Input: part model. Units: mm. Frame: model coordinates. Round coordinates to 2 decimals unless told otherwise and drop trailing zeros. Write each loop counter-clockwise with the first axis right and the second up, starting at its lowest first coordinate (ties: lowest second). Pieces come first, ordered by that corner, then holes. Notation, with made-up numbers: (-6, 40) - (29, 40) arc R12 cw to (29, 46) - close; hole circle Ø9 at (-12, 49.25). An arc over 180 degrees is marked (long way). Use one line per item in the form item = value.
Solid Edge part; units mm, degrees
sketch "Sketch1" plane through (0, 0, 0) normal (1, 0, 0) x (0, 1, 0)
  circle A0 centre (0, 0) radius 5
extrude "Protrusion1" add sketch "Sketch1" along normal mid plane 55
cosmetic_thread "Thread_1" thread depth 15
cosmetic_thread "Thread_2" thread depth 18
sketch "Sketch2" plane through (0, 0, 0) normal (0, 0, 1) x (1, 0, 0)
  circle A0 centre (-23.5, 0) radius 1.4
  circle A1 centre (23.5, 0) radius 1.25
extrude "ExtrudedCutout_1" cut sketch "Sketch2" along normal mid plane 31.5098
(1) Draft query along X for faces 1 (the face through (-27.5, 0, 0)), 2 (the face through (27.5, 0, 0)), 3 (the face through (24.655, 0.479, -0.07)). Return one class per face: released by +X, released by -X, zero draft, split by the parting line, or undercut.
Derived:
face_1 = released by -X
face_2 = released by +X
face_3 = undercut
(2) Cut plane D-D on x = -8. Output: boundary loops of the cut face in (y, z).
Derived:
outline = circle Ø10 at (0, 0)
(3) First-contact query: pin 1 Ø1.5 at (x, y) = (3.5, -2) entering from -Z; pin 2 Ø6 at (x, y) = (5.5, -3) entering from +Z; pin 3 Ø1.5 at (x, z) = (-12, -2.5) entering from -Y; pin 4 Ø3 at (x, y) = (-19, 2.5) entering from +Z. Flat tips, straight axial feed; report the tip coordinate or a pass-through.
Derived:
pin_1 = -4.84
pin_2 = 5
pin_3 = -4.68
pin_4 = 4.9
(4) Cut plane B-B on z = 0. Output: boundary loops of the cut face in (x, y).
Derived:
outline = (-27.5, -5) - (27.5, -5) - (27.5, 5) - (-27.5, 5) - close; hole circle Ø2.8 at (-23.5, 0); hole circle Ø2.5 at (23.5, 0)
(5) Cut plane A-A on y = 0. Output: boundary loops of the cut face in (x, z), then the cut area to 3 significant figures.
Derived:
outline = (-27.5, -5) - (-24.9, -5) - (-24.9, 5) - (-27.5, 5) - close; (-22.1, -5) - (22.25, -5) - (22.25, 5) - (-22.1, 5) - close; (24.75, -5) - (27.5, -5) - (27.5, 5) - (24.75, 5) - close
area = 497 mm^2
(6) Cut plane C-C on x = -23.5. Output: boundary loops of the cut face in (y, z).
Derived:
outline = (-1.4, -4.8) - (-1.4, 4.8) arc R5 ccw to start; (1.4, -4.8) arc R5 ccw to (1.4, 4.8) - close
(7) Material intervals for L1, parallel to X at y = 0, z = 0.25; L2, parallel to X at y = -1, z = 1; L3, parallel to Y at x = 23.5, z = -1, sorted ascending.
Derived:
L1 = -27.5 to -24.9, -22.1 to 22.25, 24.75 to 27.5
L2 = -27.5 to -24.48, -22.52 to 22.75, 24.25 to 27.5
L3 = -4.9 to -1.25, 1.25 to 4.9
